For this review, take the finished solid that the model builds, in its own axes (mm). Round coordinates to 2 decimals unless told otherwise and drop trailing zeros. Write each loop counter-clockwise with the first axis right and the second up, starting at its lowest first coordinate (ties: lowest second). Pieces come first, ordered by that corner, then holes. Notation, with made-up numbers: (-26.75, -31.75) - (32.25, -31.75) arc R30 ccw to (32.25, 5.25) - close; hole circle Ø11 at (-36, 71). An arc over 180 degrees is marked (long way). Answer in a Markdown table with one row per item. Add a question column.
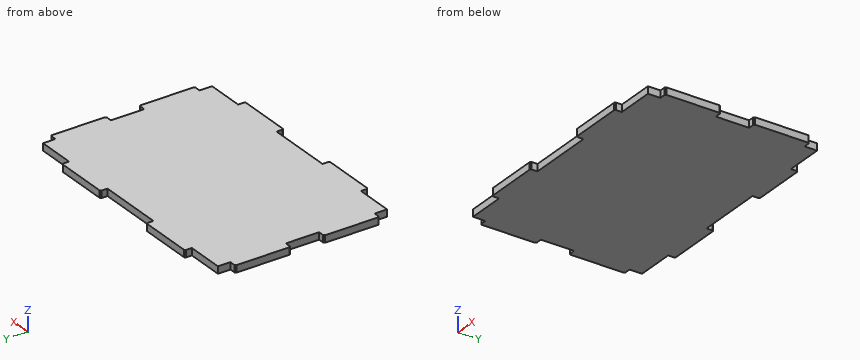
from build123d import *

# Parameters (mm, degrees)
F1_DEPTH = 12.7
F2_SIZE  = 2


with BuildPart() as f1:
    # F0 (on Top) → F1 (new body)
    with BuildSketch(Plane.XY):
        Polygon((160, -152.5), (228, -152.5), (228, -130), (240.7, -130), (240.7, -30), (228, -30), (228, 30), (240.7, 30), (240.7, 130), (228, 130), (228, 152.5), (160, 152.5), (160, 165.2), (60, 165.2), (60, 152.5), (-60, 152.5), (-60, 165.2), (-160, 165.2), (-160, 152.5), (-228, 152.5), (-228, 130), (-240.7, 130), (-240.7, 30), (-228, 30), (-228, -30), (-240.7, -30), (-240.7, -130), (-228, -130), (-228, -152.5), (-160, -152.5), (-160, -165.2), (-60, -165.2), (-60, -152.5), (60, -152.5), (60, -165.2), (160, -165.2), align=None)
    extrude(amount=F1_DEPTH)

    # F2
    f2_edges = [f1.edges().sort_by_distance(p)[0] for p in [
        (160, 165.2, 6.35),
        (240.7, 130, 6.35),
        (240.7, 30, 6.35),
        (240.7, -30, 6.35),
        (240.7, -130, 6.35),
        (160, -165.2, 6.35),
        (-60, 165.2, 6.35),
        (60, 165.2, 6.35),
        (-160, 165.2, 6.35),
        (60, -165.2, 6.35),
        (-60, -165.2, 6.35),
        (-160, -165.2, 6.35),
        (-240.7, -130, 6.35),
        (-240.7, -30, 6.35),
        (-240.7, 30, 6.35),
        (-240.7, 130, 6.35),
    ]]
    chamfer(f2_edges, length=F2_SIZE)


solid = f1.part
Q1. Insertion check: pin 1 Ø5.5 at (x, z) = (232.5, 6.5) entering from -Y; pin 2 Ø4 at (x, z) = (-207, 7) entering from -Y; pin 3 Ø3 at (y, z) = (10, 8) entering from +X. Each pin has a flat end and moves straight along its axis. Give the tip position at first contact, or say it passes through.
Q2. Add section A-A on x = 211. State the section outline as (y, z) points, then the cut area to 3 significant figures.
Q3. To check wall thickness, follow probe 1 along X at (y, z) = (-11.5, 12.25); probe 2 along Y at (x, z) = (195, 8). State the ranges of each line that lie inside material, in increasing order.
Answer sheet:
| question | item | result |
|---|---|---|
| 1 | pin 1 | stops at y = -130 |
| 1 | pin 2 | stops at y = -152.5 |
| 1 | pin 3 | stops at x = 228 |
| 2 | outline | (-152.5, 0) - (152.5, 0) - (152.5, 12.7) - (-152.5, 12.7) - close |
| 2 | area | 3,870 mm² |
| 3 | probe 1 | x = -228 to 228 |
| 3 | probe 2 | y = -152.5 to 152.5 |
